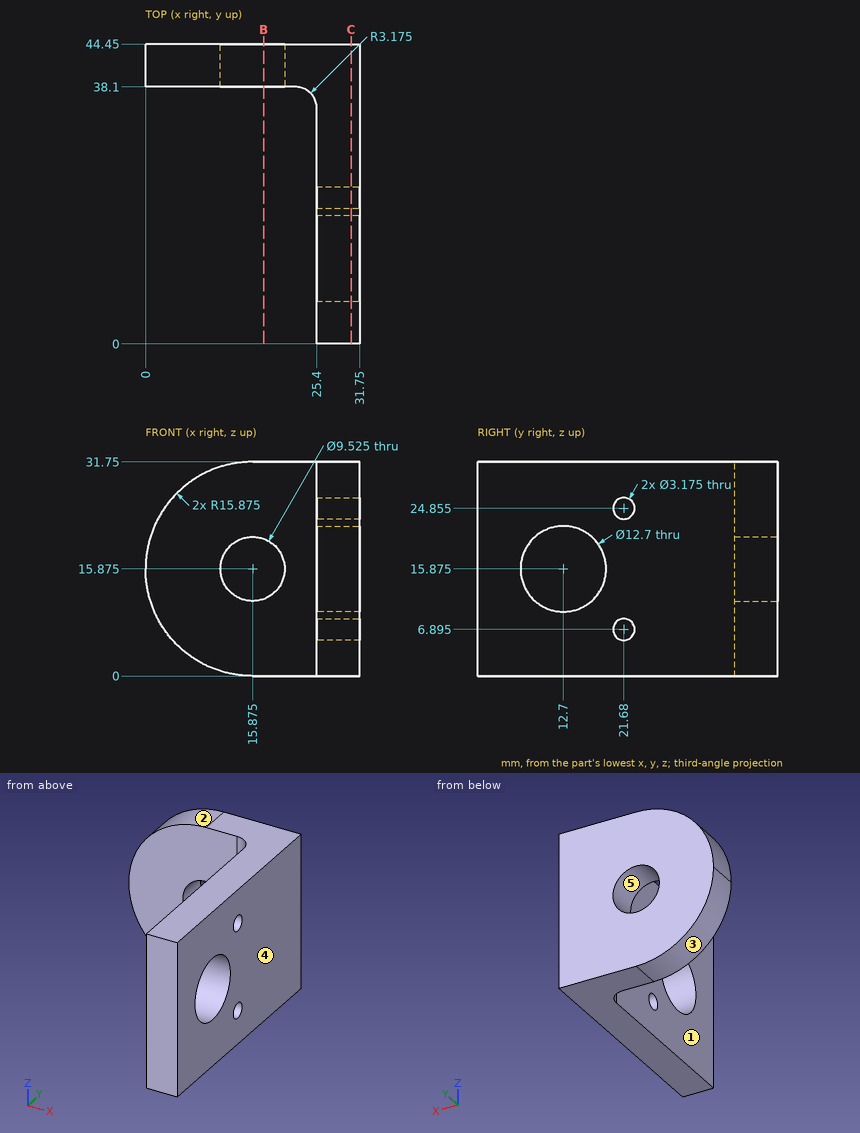
Answer from the drawing. Dimensions are ordinates in mm from the lowest x, y and z of the part. A direction names the side the tool comes from. Round coordinates to 2 decimals unless told otherwise and drop trailing zeros. Loops run counter-clockwise (first coordinate to the right, second up) from the corner with the lowest first, then second, coordinate; pieces in that order, holes last.
1) A cutting plane is placed at B-B on x = 17.5. Determine the outline of the cut face in (y, z), plus the area to 3 significant figures.
Outcome:
outline: (38.1, 0) - (44.45, 0) - (44.45, 11.4) - (38.1, 11.4) - close; (38.1, 20.35) - (44.45, 20.35) - (44.45, 31.75) - (38.1, 31.75) - close
area: 145 mm2
2) Consider line 1 (Y direction, x = 20.5, z = 21); line 2 (X direction, y = 9, z = 22.5); line 3 (Z direction, x = 26.5, y = 21). Determine where each line is inside the solid, lowest interval first.
Outcome:
line 1: y = 38.1 to 44.45
line 2: x = 25.4 to 31.75
line 3: z = 0 to 5.46, 8.33 to 23.42, 26.29 to 31.75
3) Given P1, Ø12, axis at x = 13.5, z = 4.5, coming from the -Y side; P2, Ø5, axis at y = 21.68, z = 24.86, coming from the +X side; P3, Ø12, axis at x = 6, y = 34, coming from the -Z side; P4, Ø11.5, axis at y = 12.7, z = 15.875, coming from the +X side, each flat-ended and moving along its own axis, determine where each tip first touches the part or whether it passes through.
Outcome:
P1: stops at y = 38.1
P2: stops at x = 31.75
P3: stops at z = 0.98
P4: passes through
4) A cutting plane is placed at C-C on x = 30.5. Give the number of separate pieces and of enclosed holes in the cut face, plus the area to 3 significant figures.
Outcome:
separate pieces: 1
enclosed holes: 3
area: 1,270 mm2
5) For the marked faces 1 and 2, determine the directions among +Z, -Z, +X, -X, +Y, -Y from which every point of the face is accessible in a straight line to the end or side of a thin tool.
Outcome:
face 1: +Z, -Z, -X, -Y
face 2: +Z, -X, +Y, -Y
6) For a pull along X with two mould halves and no side action, classify the marked faces 3, 4 and 5 as released by +X, released by -X, zero draft, split by the parting line, or undercut.
Outcome:
face 3: released by -X
face 4: released by +X
face 5: undercut
